```python
from build123d import *

# Parameters (mm, degrees)
SKETCH1_R           = 11.5
SKETCH1_R_2         = 9
BOSS_EXTRUDE1_DEPTH = 3.5


with BuildPart() as part:
    # Sketch1 → Boss-Extrude1 (new body)
    # profile 1 of 4: a face of its own
    with BuildSketch(Plane.XY):
        Circle(SKETCH1_R)
        Circle(SKETCH1_R_2, mode=Mode.SUBTRACT)
    # profile 2 of 4: a face of its own
    with BuildSketch(Plane.XY):
        with BuildLine():
            Line((1.75, 5.739120142), (1.75, 8.828221792))
            ThreePointArc((1.75, 8.828221792), (0, 9), (-1.75, 8.828221792))
            Line((-1.75, 8.828221792), (-1.75, 5.739120142))
            ThreePointArc((-1.75, 5.739120142), (0, 6), (1.75, 5.739120142))
        make_face()
    # profile 3 of 4: a face of its own
    with BuildSketch(Plane.XY):
        with BuildLine():
            ThreePointArc((-8.520464342, -2.898566439), (-7.794228634, -4.5), (-6.770464342, -5.929655352))
            Line((-6.770464342, -5.929655352), (-4.095223838, -4.385104527))
            ThreePointArc((-4.095223838, -4.385104527), (-5.196152423, -3), (-5.845223838, -1.354015614))
            Line((-5.845223838, -1.354015614), (-8.520464342, -2.898566439))
        make_face()
    # profile 4 of 4: a face of its own
    with BuildSketch(Plane.XY):
        with BuildLine():
            ThreePointArc((6.770464342, -5.929655352), (7.794228634, -4.5), (8.520464342, -2.898566439))
            Line((8.520464342, -2.898566439), (5.845223838, -1.354015614))
            ThreePointArc((5.845223838, -1.354015614), (5.196152423, -3), (4.095223838, -4.385104527))
            Line((4.095223838, -4.385104527), (6.770464342, -5.929655352))
        make_face()
    extrude(amount=BOSS_EXTRUDE1_DEPTH)


solid = part.part
```
Could you check a few things on this model? Use its own coordinates, in mm. A direction names the side the tool comes from. Give positions to 0.01 mm unless a question says otherwise; leave off trailing zeros. Write each loop counter-clockwise with the first axis right and the second up, starting at its lowest first coordinate (ties: lowest second). Pieces come first, ordered by that corner, then holes. Notation, with made-up numbers: (16.25, 43.5) -> (46.25, 43.5) arc R24 ccw to (46.25, 62.5) -> close; hole circle Ø7 at (56, 30.5). An arc over 180 degrees is marked (long way). Write each question's results on one line, items separated by ' | '.
1. I want a section at A-A, the plane y = 0. Write out the boundary of the cut face in (x, z).
Check sheet entries:
outline: (-11.5, 0) -> (-9, 0) -> (-9, 3.5) -> (-11.5, 3.5) -> close; (9, 0) -> (11.5, 0) -> (11.5, 3.5) -> (9, 3.5) -> close
2. I need wall thicknesses on L1, parallel to Y at x = -5.5, z = 3.45; L2, parallel to X at y = -2.5, z = 2.65; L3, parallel to Y at x = 6.5, z = 1.3. Which ranges of each line are inside material? Lowest first, please.
Check sheet entries:
L1: y = -10.1 to -7.12, -5.2 to -2.4, 7.12 to 10.1 | L2: x = -11.22 to -8.65, -7.83 to -5.45, 5.45 to 7.83, 8.65 to 11.22 | L3: y = -9.49 to -6.22, -5.77 to -1.73, 6.22 to 9.49
3. I want a section at C-C, the plane z = 2.1. Write out the boundary of the cut face in (x, y), then the cut area to 3 significant figures.
Check sheet entries:
outline: circle Ø23 at (0, 0); hole (-8.52, -2.9) -> (-5.85, -1.35) arc R6 ccw to (-4.1, -4.39) -> (-6.77, -5.93) arc R9 ccw to (6.77, -5.93) -> (4.1, -4.39) arc R6 ccw to (5.85, -1.35) -> (8.52, -2.9) arc R9 ccw to (1.75, 8.83) -> (1.75, 5.74) arc R6 ccw to (-1.75, 5.74) -> (-1.75, 8.83) arc R9 ccw to start | area: 193 mm²
4. Will these pins go through, and if not, where does the flat tip stop? pin 1 Ø1.5 at (x, y) = (-2.5, 4) entering from -Z; pin 2 Ø1.5 at (y, z) = (7, 1) entering from +X.
Check sheet entries:
pin 1: passes through | pin 2: stops at x = 9.65
5. On a 3-axis mill with a long thin cutter (end or side, diameter ignored), from which of +Z, -Z, +X, -X, +Y, -Y can I reach the whole of each face in a straight line? I mean faces 4 (the cylindrical face through (5.209, -2.978, 1.726)), 5 (the flat face through (0, 8, 0)). Say none if no direction works.
Check sheet entries:
face 4: +Z, -Z | face 5: -Z, +X, -X, +Y, -Y
6. I want a section at B-B, the plane x = 0. Write out the boundary of the cut face in (y, z), then the cut area to 3 significant figures.
Check sheet entries:
outline: (-11.5, 0) -> (-9, 0) -> (-9, 3.5) -> (-11.5, 3.5) -> close; (6, 0) -> (11.5, 0) -> (11.5, 3.5) -> (6, 3.5) -> close | area: 28.0 mm²
7. I want a section at D-D, the plane y = 10.25. Write out the boundary of the cut face in (x, z), then the cut area to 3 significant figures.
Check sheet entries:
outline: (-5.21, 0) -> (5.21, 0) -> (5.21, 3.5) -> (-5.21, 3.5) -> close | area: 36.5 mm²
8. If we mould it in two halves opening along Y, with no side actions, what happens to faces 1 (the cylindrical face through (0, -9, 2)), 2 (the flat face through (0, 8, 3.5)), 3 (the cylindrical face through (-1.5, 11.4, 1.7))? For each: released by +Y, released by -Y, zero draft, split by the parting line, or undercut.
Check sheet entries:
face 1: undercut | face 2: zero draft | face 3: split by the parting line
